Verification items for the finished model (mm, model axes). A direction names the side the tool comes from. Coordinates: 2 decimals unless noted, no trailing zeros. Order: outer loops, then holes, each group sorted by start corner. A loop starts at its lowest first (then second) coordinate and runs counter-clockwise, first axis right, second up.
Q1. Cross-section at A-A, the plane x = 55.5. Record the boundary of the cut face in (y, z).
Q2. Thickness scan on line 1 (Z direction, x = -33, y = -2.7); line 2 (X direction, y = -2.6, z = 8); line 3 (Z direction, x = 32.5, y = -1.15). Record the ranges inside material, lowest first.
Q3. Draft check along Z on faces 1 (the flat face through (-36.17, -1.48, -0.43)), 2 (the flat face through (97.89, -1.48, 3.83)), 3 (the flat face through (2, -3, 0)). Enter one of: pulls with the +Z half, pulls with the -Z half, needs draft (parallel to the pull), parting line crosses it, or undercut.
Q4. Depth check by flat-ended pin: P1, Ø0.9, axis at y = -1, z = -1, coming from the +X side. Enter the tip coordinate at first touch or a pass-through.
Q5. Cross-section at B-B, the plane y = -0.5. Count the separate pieces of the cut face and the enclosed holes in it, and give its area (3 significant figures).
Q6. Set-up check for faces 4 (the flat face through (-61.46, -1.48, -1.94)), 5 (the flat face through (2, 0, 0)): record each of +Z, -Z, +X, -X, +Y, -Y from which the full face is reachable in a straight line by a thin tool's end or side.
from build123d import *

# Parameters (mm, degrees)
F1_DEPTH = 3


# Not quite as in the source:
# - ends of sketch curves that miss each other by under 0.0002 mm in the source are joined


with BuildPart() as f1:
    # F0 (on Front) → F1 (new body)
    with BuildSketch(Plane.XZ):
        Polygon((-0.0539638903, 18.370702), (-0.0038508903, -18.362152), (92.7633391097, -18.370702), (92.6924631097, -15.890233), (103.1813041097, -16.102845), (107.7170111097, -11.141907), (106.5122111097, -7.173158), (104.2443611097, -2.991796), (101.0845361097, 1.130854), (94.6101381097, 6.599435), (89.0528781097, 9.821526), (83.6210411097, 12.103627), (77.1418581097, 13.991338), (65.1238321097, 15.930635), (57.6115531097, 16.922822), (45.9973841097, 17.743913), (32.1186031097, 18.070024), (13.3763291097, 18.270477), align=None)
        with BuildLine():
            add(Edge.make_bspline(
                [(65.6943371097, -12.899831), (62.5550341097, -12.172951), (61.7713101097, -8.692501), (64.1909471097, -7.08672)],
                knots=[0, 0, 0, 0, 1, 1, 1, 1], degree=3))
            Line((64.1909471097, -7.08672), (82.7828791097, 5.441539))
            add(Edge.make_bspline(
                [(82.7828791097, 5.441539), (83.8783131097, 5.841711), (85.0121781097, 5.972881), (86.2406861097, 5.441541)],
                knots=[0, 0, 0, 0, 1, 1, 1, 1], degree=3))
            add(Edge.make_bspline(
                [(86.2406861097, 5.441541), (88.5854111097, 4.25464), (90.9595961097, 3.079519), (92.6551511097, 1.632949)],
                knots=[0, 0, 0, 0, 1, 1, 1, 1], degree=3))
            add(Edge.make_bspline(
                [(92.6551511097, 1.632949), (93.7989981097, 0.505006), (94.7332961097, -0.581922), (95.6118231097, -1.97519)],
                knots=[0, 0, 0, 0, 1, 1, 1, 1], degree=3))
            add(Edge.make_bspline(
                [(95.6118231097, -1.97519), (95.8557461097, -3.177903), (96.2772981097, -4.480841), (96.2632881097, -5.683554)],
                knots=[0, 0, 0, 0, 1, 1, 1, 1], degree=3))
            add(Edge.make_bspline(
                [(96.2632881097, -5.683554), (95.9762411097, -6.899896), (95.9073311097, -8.384491), (95.3612561097, -9.341805)],
                knots=[0, 0, 0, 0, 1, 1, 1, 1], degree=3))
            add(Edge.make_bspline(
                [(95.3612561097, -9.341805), (94.8500481097, -10.267174), (94.1296281097, -10.933218), (93.3567311097, -11.596892)],
                knots=[0, 0, 0, 0, 1, 1, 1, 1], degree=3))
            add(Edge.make_bspline(
                [(93.3567311097, -11.596892), (92.4958131097, -12.139141), (91.1271531097, -12.72489), (89.9991611097, -13.000059)],
                knots=[0, 0, 0, 0, 1, 1, 1, 1], degree=3))
            Line((89.9991611097, -13.000059), (65.6943371097, -12.899831))
        make_face(mode=Mode.SUBTRACT)
        with BuildLine():
            Line((3.8548531097, -8.790562), (3.8548531097, 9.450582))
            add(Edge.make_bspline(
                [(10.8706771097, 11.755782), (8.5680291097, 13.13931), (5.1563371097, 13.150107), (3.8548531097, 9.450582)],
                knots=[0, 0, 0, 0, 1, 1, 1, 1], degree=3))
            Line((10.8706771097, 11.755782), (36.1276481097, -7.28717))
            add(Edge.make_bspline(
                [(32.9204121097, -12.799606), (35.7071221097, -12.751328), (37.1961481097, -10.572453), (36.1276481097, -7.28717)],
                knots=[0, 0, 0, 0, 1, 1, 1, 1], degree=3))
            Line((32.9204121097, -12.799606), (7.5632171097, -12.899831))
            add(Edge.make_bspline(
                [(3.8548531097, -8.790562), (3.7573371097, -11.04941), (4.4717691097, -12.766958), (7.5632171097, -12.899831)],
                knots=[0, 0, 0, 0, 1, 1, 1, 1], degree=3))
        make_face(mode=Mode.SUBTRACT)
        with BuildLine():
            Line((45.9498021097, -7.788301), (26.1050401097, 7.145382))
            add(Edge.make_bspline(
                [(29.7131791097, 12.657816), (26.6289141097, 12.752098), (24.0319891097, 10.480568), (26.1050401097, 7.145382)],
                knots=[0, 0, 0, 0, 1, 1, 1, 1], degree=3))
            Line((29.7131791097, 12.657816), (49.0586381097, 11.882658))
            Line((49.0586381097, 11.882658), (68.4505551097, 10.001826))
            add(Edge.make_bspline(
                [(70.2045121097, 3.938149), (72.7849811097, 5.68209), (72.6619441097, 8.999483), (68.4505551097, 10.001826)],
                knots=[0, 0, 0, 0, 1, 1, 1, 1], degree=3))
            Line((70.2045121097, 3.938149), (52.4644981097, -7.988753))
            add(Edge.make_bspline(
                [(45.9498021097, -7.788301), (47.6692371097, -9.607126), (49.6811001097, -10.292787), (52.4644981097, -7.988753)],
                knots=[0, 0, 0, 0, 1, 1, 1, 1], degree=3))
        make_face(mode=Mode.SUBTRACT)
    extrude(amount=F1_DEPTH)

    # F2: F1 across plane


with BuildPart() as f1_1:
    add(f1.part)
    add(f1.part.mirror(Plane.YZ))


solid = f1_1.part
Check values:
1. outline: (-3, -18.37) - (0, -18.37) - (0, -5.95) - (-3, -5.95) - close; (-3, 11.26) - (0, 11.26) - (0, 17.07) - (-3, 17.07) - close
2. line 1: z = -18.37 to -12.8, -4.93 to 1.96, 12.53 to 18.05
2. line 2: x = -92.19 to -71.6, -25.66 to -15.85, -3.85 to 3.85, 15.85 to 25.66, 71.6 to 92.19
2. line 3: z = -18.37 to -12.8, -4.55 to 2.33, 12.55 to 18.06
3. face 1: undercut
3. face 2: pulls with the +Z half
3. face 3: needs draft
4. P1: stops at x = 103.06
5. separate pieces: 1
5. enclosed holes: 6
5. area: 3,710 mm2
6. face 4: +Y, -Y
6. face 5: +Z, -Z, +X, -X, +Y
